Print and shaded views of the part. All mm, measured from the part's lowest x, y and z. Round coordinates to 2 decimals unless told otherwise and drop trailing zeros. Loops run counter-clockwise (first coordinate to the right, second up) from the corner with the lowest first, then second, coordinate; pieces in that order, holes last. Notation, with made-up numbers: (-17.75, 2) - (41.25, 2) arc R5 cw to (41.25, 11) - close; hole circle Ø6 at (29.25, 43.5). An arc over 180 degrees is marked (long way). Use one line per item in the form item = value.
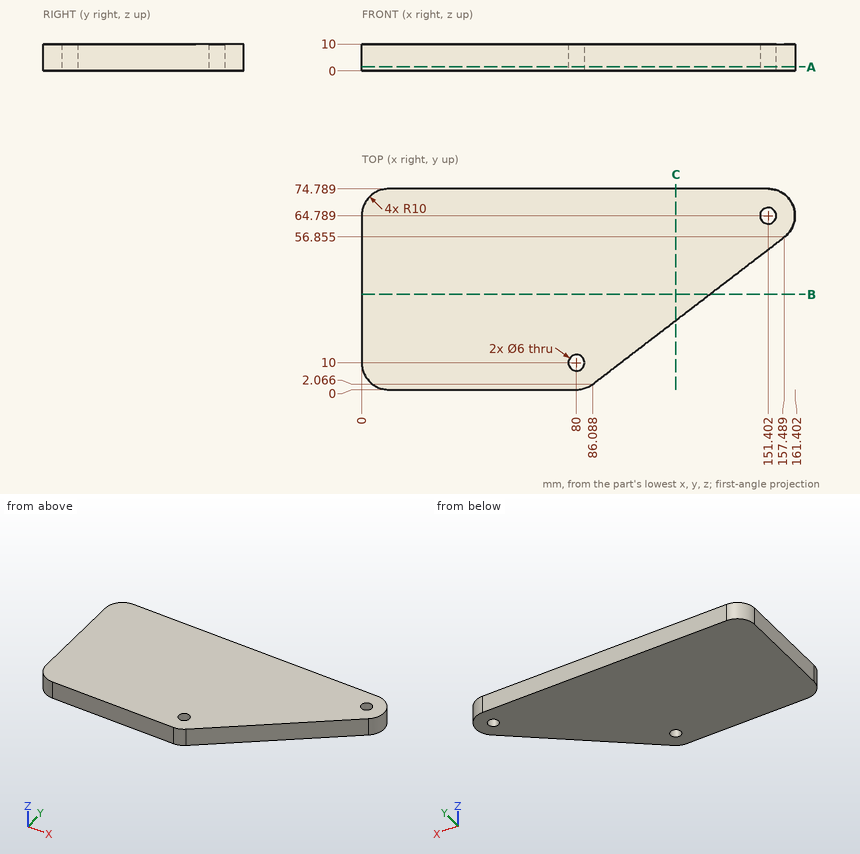
1) Slice it at C-C (x = 117). Write the cut outline in (y, z), plus the area to 3 significant figures.
Report:
outline = (25.79, 0) - (74.79, 0) - (74.79, 10) - (25.79, 10) - close
area = 490 mm^2
2) Drill centre lines: probe 1 along Y at (x, z) = (80, 2.25); probe 2 along X at (y, z) = (12, 8.25) (1 decimal); probe 3 along X at (y, z) = (20.5, 4). Where is each one in solid material? Low to high.
Report:
probe_1 = 0 to 7, 13 to 74.79
probe_2 = 0 to 77.8, 82.2 to 99
probe_3 = 0 to 110.11
3) Flat gauge pins, fed straight in: pin 1 (5.5 mm diameter, centred on x = 80, y = 10, fed in from -Z); pin 2 (3 mm diameter, centred on x = 142.5, z = 9, fed in from -Y). Where does each tip first touch, or does it go through?
Report:
pin_1 = through
pin_2 = 44.2
4) Slice it at B-B (y = 35.5). Write the cut outline in (x, z).
Report:
outline = (0, 0) - (129.66, 0) - (129.66, 10) - (0, 10) - close
5) Slice it at A-A (z = 1.5). Write the cut outline in (x, y) (1 decimal).
Report:
outline = (0, 10) arc R10 ccw to (10, 0) - (80, 0) arc R10 ccw to (86.1, 2.1) - (157.5, 56.9) arc R10 ccw to (151.4, 74.8) - (10, 74.8) arc R10 ccw to (0, 64.8) - close; hole circle Ø6 at (80, 10); hole circle Ø6 at (151.4, 64.8)
